Verification items for the finished model (mm, model axes). A direction names the side the tool comes from. Coordinates: 2 decimals unless noted, no trailing zeros. Write each loop counter-clockwise with the first axis right and the second up, starting at its lowest first coordinate (ties: lowest second). Pieces come first, ordered by that corner, then holes. Notation, with made-up numbers: (63.25, 70) - (84.25, 70) arc R35 cw to (84.25, 103) - close; hole circle Ø1 at (64, 16). An arc over 180 degrees is marked (long way). Use CSV: the item, a comma, the result in double quotes. Start each with the question number.
Autodesk Inventor part; units mm, degrees
ref_plane "YZ Plane" through (0, 0, 0) normal (1, 0, 0) x (0, 1, 0)
ref_plane "XZ Plane" through (0, 0, 0) normal (0, 1, 0) x (-1, 0, 0)
ref_plane "XY Plane" through (0, 0, 0) normal (0, 0, 1) x (1, 0, 0)
sketch "Esquisse1" plane through (0, 0, 0) normal (0, 0, 1) x (1, 0, 0)
  circle A0 centre (0, 0) radius 40
  circle A1 centre (0, 0) radius 6
  line L0 (0, 0) -> (16, 0) construction
  circle A2 centre (0, 0) radius 16 construction
  line L1 (6, 0) -> (16, 0) construction
  line L2 (0, 0) -> (0, 28) construction
  circle A3 centre (0, 28) radius 2
  circle A4 centre (-28, 0) radius 2
  circle A5 centre (0, -28) radius 2
  circle A6 centre (28, 0) radius 2
  dimension "d1" = 12
  dimension "d0" = 80
  dimension "d3" = 10
  dimension "d5" = 4
  dimension "d6" = 28
  dimension "d9" = 360
extrude "Extrusion1" add sketch "Esquisse1" along normal blind 29
sketch "Esquisse2" plane through (0, 0, 29) normal (0, 0, 1) x (1, 0, 0)
  circle A0 centre (0, 0) radius 6
  circle A1 centre (0, 0) radius 40
  line L0 (0, 0) -> (6, 0) construction
  line L1 (6, 0) -> (16, 0) construction
  circle A2 centre (0, 0) radius 16
  dimension "d15" = 10
extrude "Extrusion2" cut sketch "Esquisse2" against normal blind 10 contours A2
sketch "Esquisse3" plane through (0, 0, 0) normal (0, 0, -1) x (-1, 0, 0)
  circle A0 centre (0, 0) radius 6
  circle A1 centre (-28, 0) radius 2
  circle A2 centre (0, -28) radius 2
  circle A3 centre (28, 0) radius 2
  circle A4 centre (0, 28) radius 2
  circle A5 centre (0, 0) radius 40
  line L0 (3.5, 25.9793) -> (0, 23.9585)
  line L1 (0, 23.9585) -> (-3.5, 25.9793)
  line L2 (-3.5, 25.9793) -> (-3.5, 30.0207)
  line L3 (-3.5, 30.0207) -> (0, 32.0415)
  line L4 (0, 32.0415) -> (3.5, 30.0207)
  line L5 (3.5, 30.0207) -> (3.5, 25.9793)
  line L6 (-3.5, 25.9793) -> (3.5, 25.9793) construction
  line L7 (0, 0) -> (0, -40) construction
  line L8 (-25.9793, 3.5) -> (-23.9585, 0)
  line L9 (-23.9585, 0) -> (-25.9793, -3.5)
  line L10 (-25.9793, -3.5) -> (-30.0207, -3.5)
  line L11 (-30.0207, -3.5) -> (-32.0415, 0)
  line L12 (-32.0415, 0) -> (-30.0207, 3.5)
  line L13 (-30.0207, 3.5) -> (-25.9793, 3.5)
  line L14 (-3.5, -25.9793) -> (0, -23.9585)
  line L15 (0, -23.9585) -> (3.5, -25.9793)
  line L16 (3.5, -25.9793) -> (3.5, -30.0207)
  line L17 (3.5, -30.0207) -> (0, -32.0415)
  line L18 (0, -32.0415) -> (-3.5, -30.0207)
  line L19 (-3.5, -30.0207) -> (-3.5, -25.9793)
  line L20 (25.9793, -3.5) -> (23.9585, 0)
  line L21 (23.9585, 0) -> (25.9793, 3.5)
  line L22 (25.9793, 3.5) -> (30.0207, 3.5)
  line L23 (30.0207, 3.5) -> (32.0415, 0)
  line L24 (32.0415, 0) -> (30.0207, -3.5)
  line L25 (30.0207, -3.5) -> (25.9793, -3.5)
  point P0 (-25.9793, 3.5)
  point P1 (-3.5, -25.9793)
  point P2 (25.9793, -3.5)
  dimension "d18" = 7
  dimension "d21" = 360
extrude "Extrusion3" cut sketch "Esquisse3" against normal blind 3 contours L0 L1 L2 L3 L4 L5 | L8 L9 L10 L11 L12 L13 | L14 L15 L16 L17 L18 L19 | L20 L21 L22 L23 L24 L25
sketch "Esquisse4" plane through (0, 0, 29) normal (0, 0, 1) x (1, 0, 0)
  circle A0 centre (0, 0) radius 16
  circle A1 centre (0, 0) radius 40
  line L0 (0, 0) -> (18.3848, 18.3848) construction
  line L1 (0, 0) -> (26, 0) construction
  circle A2 centre (18.3848, 18.3848) radius 2
  circle A3 centre (-18.3848, 18.3848) radius 2
  circle A4 centre (-18.3848, -18.3848) radius 2
  circle A5 centre (18.3848, -18.3848) radius 2
  dimension "d25" = 26
  dimension "d26" = 45
  dimension "d27" = 4
  dimension "d30" = 360
extrude "Extrusion4" cut sketch "Esquisse4" against normal through all contours A2 | A3 | A4 | A5
sketch "Esquisse5" plane through (0, 0, 29) normal (0, 0, 1) x (1, 0, 0)
  circle A0 centre (-18.3848, -18.3848) radius 2
  circle A1 centre (18.3848, 18.3848) radius 2
  circle A2 centre (-18.3848, 18.3848) radius 2
  circle A3 centre (18.3848, -18.3848) radius 2
  circle A4 centre (0, 0) radius 16
  circle A5 centre (0, 0) radius 40
  line L0 (14.8848, 16.3641) -> (14.8848, 20.4055)
  line L1 (14.8848, 20.4055) -> (18.3848, 22.4262)
  line L2 (18.3848, 22.4262) -> (21.8848, 20.4055)
  line L3 (21.8848, 20.4055) -> (21.8848, 16.3641)
  line L4 (21.8848, 16.3641) -> (18.3848, 14.3433)
  line L5 (18.3848, 14.3433) -> (14.8848, 16.3641)
  line L6 (0, 0) -> (0, 40) construction
  line L7 (14.8848, 16.3641) -> (21.8848, 16.3641) construction
  line L8 (-16.3641, 14.8848) -> (-20.4055, 14.8848)
  line L9 (-20.4055, 14.8848) -> (-22.4262, 18.3848)
  line L10 (-22.4262, 18.3848) -> (-20.4055, 21.8848)
  line L11 (-20.4055, 21.8848) -> (-16.3641, 21.8848)
  line L12 (-16.3641, 21.8848) -> (-14.3433, 18.3848)
  line L13 (-14.3433, 18.3848) -> (-16.3641, 14.8848)
  line L14 (-14.8848, -16.3641) -> (-14.8848, -20.4055)
  line L15 (-14.8848, -20.4055) -> (-18.3848, -22.4262)
  line L16 (-18.3848, -22.4262) -> (-21.8848, -20.4055)
  line L17 (-21.8848, -20.4055) -> (-21.8848, -16.3641)
  line L18 (-21.8848, -16.3641) -> (-18.3848, -14.3433)
  line L19 (-18.3848, -14.3433) -> (-14.8848, -16.3641)
  line L20 (16.3641, -14.8848) -> (20.4055, -14.8848)
  line L21 (20.4055, -14.8848) -> (22.4262, -18.3848)
  line L22 (22.4262, -18.3848) -> (20.4055, -21.8848)
  line L23 (20.4055, -21.8848) -> (16.3641, -21.8848)
  line L24 (16.3641, -21.8848) -> (14.3433, -18.3848)
  line L25 (14.3433, -18.3848) -> (16.3641, -14.8848)
  dimension "d34" = 7
  dimension "d37" = 360
extrude "Extrusion5" cut sketch "Esquisse5" against normal blind 3 contours L0 L1 L2 L3 L4 L5 | L8 L9 L10 L11 L12 L13 | L14 L15 L16 L17 L18 L19 | L20 L21 L22 L23 L24 L25
properties part number "bowl"
Q1. Scan lines: line 1 along Y through (x, z) = (0, 11.5); line 2 along X through (y, z) = (-20, 5.5); line 3 along Y through (x, z) = (19, 10.5). Record each from-to range of solid material in increasing order. Write a range as from..to.
Q2. Release check for a two-part mould opening along X. For faces 4 (the flat face through (-28, 3.5, 1)), 5 (the flat face through (8, 1, 0)), 6 (the cylindrical face through (-19.972, 17.168, 13.182)) record: released by +X, released by -X, zero draft, split by the parting line, or undercut.
Q3. Cross-section at B-B (x = 28). Record the cut outline in (y, z), plus the area to 3 significant figures.
Q4. Cross-section at A-A (z = 23). State how many separate pieces and enclosed holes the cut face has, plus the area to 3 significant figures.
Q5. Tool access check on faces 1 (the flat face through (20.1, -16.8, 26)), 2 (the cylindrical face through (-26.092, -0.601, 15.818)), 3 (the flat face through (1.726, 24.955, 1.479)). Record the directions out of +Z, -Z, +X, -X, +Y, -Y that give a thin tool (end or side, any length) a straight path to the whole face; none if there is none.
Q6. Gauge pin test, flat ends, axial feed: pin 1 (3.5 mm diameter, centred on x = 18, z = 28, fed in from +Y); pin 2 (0.9 mm diameter, centred on x = -27.5, z = 2, fed in from +Y); pin 3 (5.5 mm diameter, centred on x = 18.5, y = -18.5, fed in from +Z). Record the tip position at first contact, or that the pin passes through.
Reply:
1,line 1,"-40..-30, -26..-6, 6..26, 30..40"
1,line 2,"-34.64..-19.56, -17.21..17.21, 19.56..34.64"
1,line 3,"-35.2..-20.29, -16.48..16.48, 20.29..35.2"
2,face 4,"undercut"
2,face 5,"zero draft"
2,face 6,"undercut"
3,outline,"(-28.57, 0) - (-3.5, 0) - (-3.5, 3) - (-2, 3) - (-2, 29) - (-28.57, 29) - close; (2, 3) - (3.5, 3) - (3.5, 0) - (28.57, 0) - (28.57, 29) - (2, 29) - close"
3,area,"1,530 mm^2"
4,separate pieces,"1"
4,enclosed holes,"9"
4,area,"4,120 mm^2"
5,face 1,"+Z"
5,face 2,"+Z, -Z"
5,face 3,"-Z"
6,pin 1,"y = 36.55"
6,pin 2,"y = 29.47"
6,pin 3,"z = 26"
